Autodesk Inventor part; units mm, degrees
ref_plane "YZ Plane" through (0, 0, 0) normal (1, 0, 0) x (0, 1, 0)
ref_plane "XZ Plane" through (0, 0, 0) normal (0, 1, 0) x (-1, 0, 0)
ref_plane "XY Plane" through (0, 0, 0) normal (0, 0, 1) x (1, 0, 0)
sketch "ExtrusionBacker_Y_350mm_B" plane through (0, 0, 0) normal (0, 0, 1) x (1, 0, 0)
  arc A0 (355.9999, 24.106) -> (357.9999, 26.106) centre (355.9999, 26.106) ccw
  line L0 (357.9999, 26.106) -> (357.9999, 40.106)
  arc A1 (357.9999, 40.106) -> (355.9999, 42.106) centre (355.9999, 40.106) ccw
  line L1 (355.9999, 42.106) -> (-30.0001, 42.106)
  arc A2 (-30.0001, 42.106) -> (-32.0001, 40.106) centre (-30.0001, 40.106) ccw
  line L2 (-32.0001, 40.106) -> (-32.0001, 26.106)
  arc A3 (-32.0001, 26.106) -> (-30.0001, 24.106) centre (-30.0001, 26.106) ccw
  line L3 (-30.0001, 24.106) -> (355.9999, 24.106)
  line L4 (322.9999, 37.0031) -> (328.736, 33.6914)
  line L5 (328.736, 33.6914) -> (328.736, 36.2894)
  line L6 (328.736, 36.2894) -> (322.9999, 39.6012)
  line L7 (322.9999, 39.6012) -> (322.9999, 37.0031)
  line L8 (317.2637, 35.1187) -> (317.2637, 37.7168)
  line L9 (317.2637, 37.7168) -> (328.736, 31.0933)
  line L10 (328.736, 31.0933) -> (328.736, 28.4952)
  line L11 (328.736, 28.4952) -> (317.2637, 35.1187)
  line L12 (317.2637, 32.5207) -> (317.2637, 29.9226)
  line L13 (317.2637, 29.9226) -> (322.9999, 26.6108)
  line L14 (322.9999, 26.6108) -> (322.9999, 29.2089)
  line L15 (322.9999, 29.2089) -> (317.2637, 32.5207)
  circle A4 centre (102.9999, 33.106) radius 1.7
  circle A5 centre (142.9999, 33.106) radius 1.7
  circle A6 centre (222.9999, 33.106) radius 1.7
  circle A7 centre (182.9999, 33.106) radius 1.7
  circle A8 centre (62.9999, 33.106) radius 1.7
  circle A9 centre (302.9999, 33.106) radius 1.7
  circle A10 centre (342.9999, 33.106) radius 1.7
  circle A11 centre (-17.0001, 33.106) radius 1.7
  circle A12 centre (22.9999, 33.106) radius 1.7
  circle A13 centre (262.9999, 33.106) radius 1.7
sketch "Skizze1" plane through (0, 0, 0) normal (0, 1, 0) x (-1, 0, 0)
  arc A0 (373, -9) -> (375, -7) centre (373, -7) ccw
  line L0 (375, -7) -> (375, 7)
  arc A1 (375, 7) -> (373, 9) centre (373, 7) ccw
  line L1 (373, 9) -> (-13, 9)
  arc A2 (-13, 9) -> (-15, 7) centre (-13, 7) ccw
  line L2 (-15, 7) -> (-15, -7)
  arc A3 (-15, -7) -> (-13, -9) centre (-13, -7) ccw
  line L3 (-13, -9) -> (373, -9)
  line L4 (340, 3.8971) -> (345.7362, 0.5853)
  line L5 (345.7362, 0.5853) -> (345.7362, 3.1834)
  line L6 (345.7362, 3.1834) -> (340, 6.4952)
  line L7 (340, 6.4952) -> (340, 3.8971)
  line L8 (334.2638, 2.0127) -> (334.2638, 4.6108)
  line L9 (334.2638, 4.6108) -> (345.7362, -2.0127)
  line L10 (345.7362, -2.0127) -> (345.7362, -4.6108)
  line L11 (345.7362, -4.6108) -> (334.2638, 2.0127)
  line L12 (334.2638, -0.5853) -> (334.2638, -3.1834)
  line L13 (334.2638, -3.1834) -> (340, -6.4952)
  line L14 (340, -6.4952) -> (340, -3.8971)
  line L15 (340, -3.8971) -> (334.2638, -0.5853)
  circle A4 centre (120, 0) radius 1.7
  circle A5 centre (160, 0) radius 1.7
  circle A6 centre (240, 0) radius 1.7
  circle A7 centre (200, 0) radius 1.7
  circle A8 centre (80, 0) radius 1.7
  circle A9 centre (320, 0) radius 1.7
  circle A10 centre (360, 0) radius 1.7
  circle A11 centre (0, 0) radius 1.7
  circle A12 centre (40, 0) radius 1.7
  circle A13 centre (280, 0) radius 1.7
  point P0 (373, -9)
  point P1 (375, 7)
  point P2 (373, 9)
  point P3 (-13, 9)
  point P4 (-15, 7)
  point P5 (-15, -7)
  point P6 (-13, -9)
  point P7 (334.2638, -0.5853)
  point P8 (340, -3.8971)
  point P9 (340, -6.4952)
  point P10 (334.2638, -3.1834)
  point P11 (334.2638, 2.0127)
  point P12 (334.2638, 4.6108)
  point P13 (345.7362, -2.0127)
  point P14 (345.7362, -4.6108)
  point P15 (340, 3.8971)
  point P16 (340, 6.4952)
  point P17 (345.7362, 0.5853)
extrude "Extrusion1" add sketch "Skizze1" along normal blind 3
sketch "Skizze2" plane through (0, 3, 0) normal (0, 1, 0) x (1, 0, 0)
  circle A0 centre (-360, 0) radius 1.7
  circle A1 centre (-320, 0) radius 1.7
  circle A2 centre (-280, 0) radius 1.7
  circle A3 centre (-240, 0) radius 1.7
  circle A4 centre (-200, 0) radius 1.7
  circle A5 centre (-160, 0) radius 1.7
  circle A6 centre (-120, 0) radius 1.7
  circle A7 centre (-80, 0) radius 1.7
  circle A8 centre (-40, 0) radius 1.7
  circle A9 centre (0, 0) radius 1.7
hole "Bohrung1" at (-360, 3, 0) at (-320, 3, 0) at (-280, 3, 0) at (-240, 3, 0) at (-200, 3, 0) at (-160, 3, 0) at (-120, 3, 0) at (-80, 3, 0) at (-40, 3, 0) at (0, 3, 0) direction (0, -1, 0) diameter 3.4 end through all countersink diameter 7.5 countersink angle 90
properties part number "Y Extrusion-Backer [B] (350mm)" material "Titan"
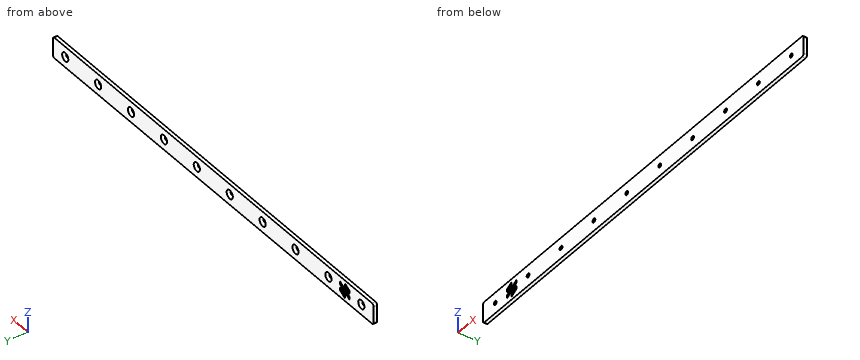
Source: CAD feature listing. Evaluate the final solid. Frame: model axes, mm. Round coordinates to 2 decimals unless told otherwise and drop trailing zeros.
Q1. Ray query, line 1 (Z direction, x = -320, y = 0.65); line 2 (X direction, y = 1.75, z = -3); line 3 (X direction, y = 0.9, z = 4.5). Return the intervals inside material, ascending.
Q2. First-contact query: P1, Ø4, axis at x = -320, z = 0, coming from the +Y side; P2, Ø5, axis at x = -269, z = 6.5, coming from the -Y side. Flat tips, straight axial feed; report the tip coordinate or a pass-through.
Q3. Section A-A, the plane y = 0.45. State how many separate pieces and enclosed holes the cut face has, plus the area to 3 significant figures.
Solutions:
1. line 1: z = -9 to -1.7, 1.7 to 9
1. line 2: x = -375 to -345.74, -342.95 to -338.45, -334.26 to 15
1. line 3: x = -375 to -343.46, -340 to -334.46, -334.26 to 15
2. P1: stops at y = 1.25
2. P2: stops at y = 0
3. separate pieces: 1
3. enclosed holes: 13
3. area: 6,870 mm2
